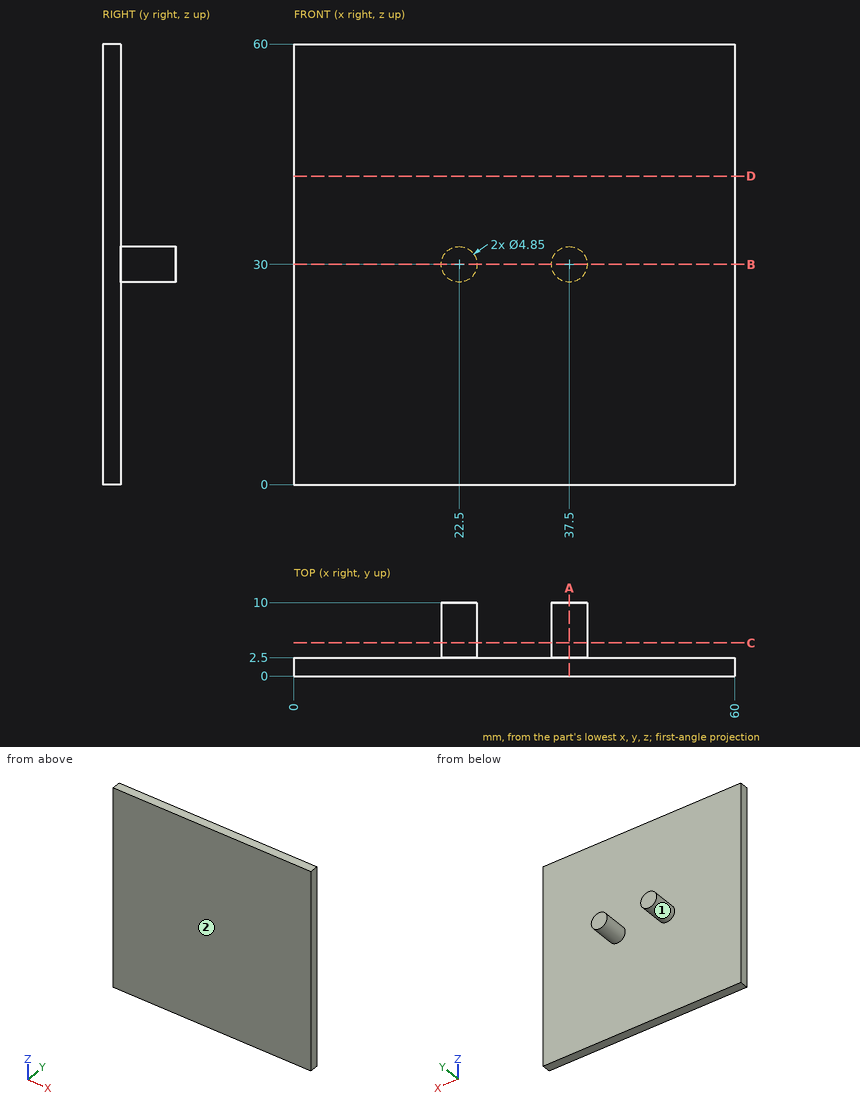
Answer from the drawing. Dimensions are ordinates in mm from the lowest x, y and z of the part. Give positions to 0.01 mm unless a question says otherwise; leave off trailing zeros. Loops run counter-clockwise (first coordinate to the right, second up) from the corner with the lowest first, then second, coordinate; pieces in that order, holes last. Notation, with made-up numbers: (15, -16) - (73, -16) arc R11 ccw to (73, -6) - close; hole circle Ø7 at (77, 89.5). An arc over 180 degrees is marked (long way). Answer as a JSON object with one key per item and string values.
1. A cutting plane is placed at C-C (y = 4.5). Write down the section's boundary in (x, z) (3 decimals), then the cut area to 3 significant figures.
Determined:
{"outline": "circle Ø4.85 at (22.5, 30); circle Ø4.85 at (37.5, 30)", "area": "36.9 mm²"}
2. For a pull along X with two mould halves and no side action, classify the marked faces 1 and 2 as pulls with the +X half, pulls with the -X half, needs draft (parallel to the pull), parting line crosses it, or undercut.
Determined:
{"face 1": "undercut", "face 2": "needs draft"}
3. A cutting plane is placed at B-B (z = 30). Write down the section's boundary in (x, y) (3 decimals).
Determined:
{"outline": "(0, 0) - (60, 0) - (60, 2.5) - (39.925, 2.5) - (39.925, 10) - (35.075, 10) - (35.075, 2.5) - (24.925, 2.5) - (24.925, 10) - (20.075, 10) - (20.075, 2.5) - (0, 2.5) - close"}
4. A cutting plane is placed at A-A (x = 37.5). Write down the section's boundary in (y, z) (3 decimals), then the cut area to 3 significant figures.
Determined:
{"outline": "(0, 0) - (2.5, 0) - (2.5, 27.575) - (10, 27.575) - (10, 32.425) - (2.5, 32.425) - (2.5, 60) - (0, 60) - close", "area": "186 mm²"}
5. A cutting plane is placed at D-D (z = 42). Write down the section's boundary in (x, y), then the cut area to 3 significant figures.
Determined:
{"outline": "(0, 0) - (60, 0) - (60, 2.5) - (0, 2.5) - close", "area": "150 mm²"}
6. Find the intervals of material crossed by L1, parallel to Y at x = 51.5, z = 15.5; L2, parallel to X at y = 9.75, z = 30.5; L3, parallel to X at y = 8.75, z = 31.5, in increasing order. Write a range as [from, to].
Determined:
{"L1": "[0, 2.5]", "L2": "[20.13, 24.87], [35.13, 39.87]", "L3": "[20.59, 24.41], [35.59, 39.41]"}
7. Flat-ended cylindrical pins translate along their axes: pin 1 Ø6 at (y, z) = (7.5, 10.5) entering from +X; pin 2 Ø3 at (x, z) = (51.5, 6.5) entering from +Y. Find the tip coordinate at first contact, or state that the pin passes through.
Determined:
{"pin 1": "through", "pin 2": "y = 2.5"}
